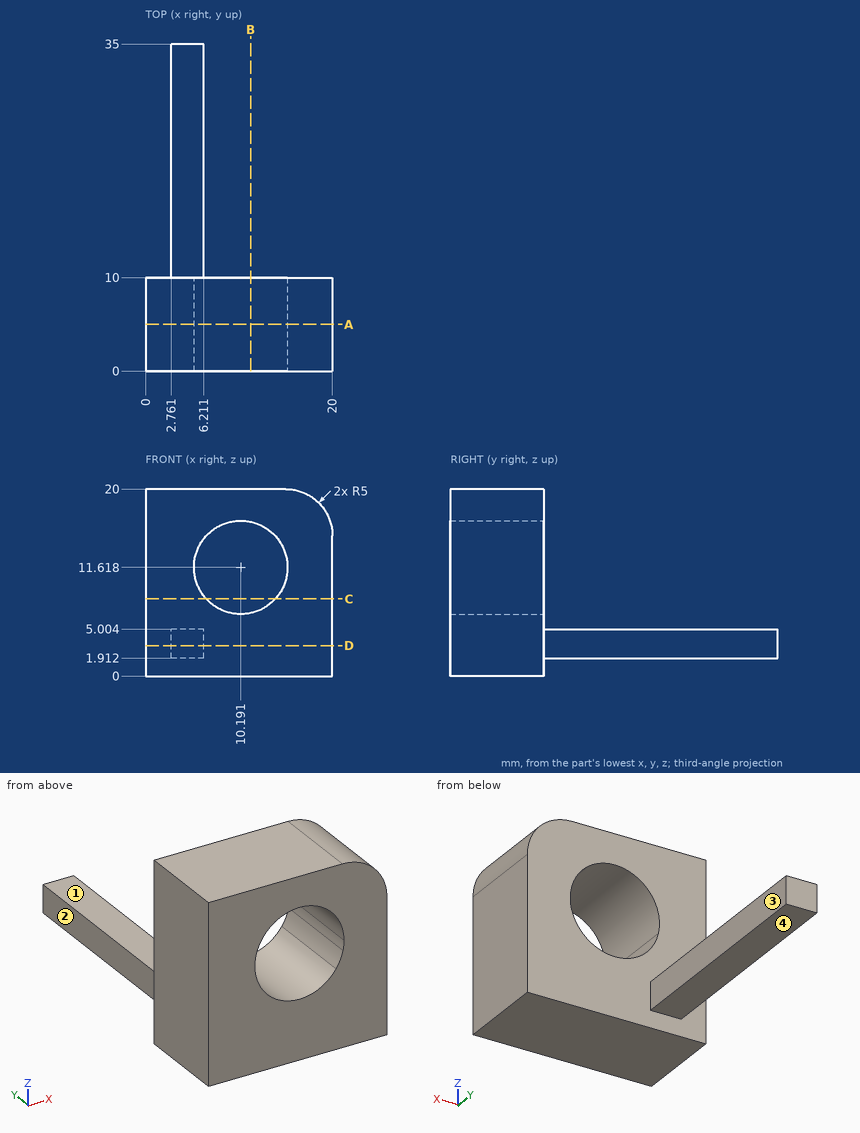
Verification items for this drawing (mm, ordinates from the low corner). A direction names the side the tool comes from. Give positions to 0.01 mm unless a question says otherwise; leave off trailing zeros. Loops run counter-clockwise (first coordinate to the right, second up) from the corner with the lowest first, then second, coordinate; pieces in that order, holes last. Notation, with made-up numbers: M -27,-27.75 L 13,-27.75 A22 ccw 13,-3.75 Z; hole C 46.5,78 d5. An arc over 180 degrees is marked long. Answer as a JSON object with one key per item and string values. Group by question number.
Item 1: Material ranges on L1, parallel to Y at x = 7, z = 3.5; L2, parallel to Z at x = 4.75, y = 22 (1 decimal); L3, parallel to X at y = 4, z = 14 (1 decimal), recorded low to high.
Item 2: Sectioned sample at D-D on z = 3.25. Record the boundary of the cut face in (x, y).
Item 3: Gauge pin test, flat ends, axial feed: pin 1 (1.5 mm diameter, centred on y = 27.5, z = 3.5, fed in from +X); pin 2 (0.9 mm diameter, centred on y = 26, z = 4, fed in from -X); pin 3 (12 mm diameter, centred on x = 9.5, z = 12.5, fed in from +Y). Record the tip position at first contact, or that the pin passes through.
Item 4: Sectioned sample at C-C on z = 8.25. Record the boundary of the cut face in (x, y) (1 decimal), plus the area to 3 significant figures.
Item 5: Access from +Z, -Z, +X, -X, +Y, -Y to the whole of each face (thin tool, end or side, straight path). Record for the marked faces 1, 2, 3 and 4.
Item 6: Sectioned sample at B-B on x = 11.25. Record the boundary of the cut face in (y, z) (1 decimal), plus the area to 3 significant figures.
Item 7: Sectioned sample at A-A on y = 5. Record the boundary of the cut face in (x, z) (1 decimal), plus the area to 3 significant figures.
Findings below:
{
 "1": {"L1": "0 to 10", "L2": "1.9 to 5", "L3": "0 to 5.8, 14.6 to 20"},
 "2": {"outline": "M 0,0 L 20,0 L 20,10 L 6.21,10 L 6.21,35 L 2.76,35 L 2.76,10 L 0,10 Z"},
 "3": {"pin 1": "x = 6.21", "pin 2": "x = 2.76", "pin 3": "y = 10"},
 "4": {"outline": "M 0,0 L 6.5,0 L 6.5,10 L 0,10 Z; M 13.9,0 L 20,0 L 20,10 L 13.9,10 Z", "area": "126 mm2"},
 "5": {"face 1": "+Z, +X, -X, +Y", "face 2": "+Z, -Z, -X, +Y", "face 3": "+Z, -Z, +X, +Y", "face 4": "-Z, +X, -X, +Y"},
 "6": {"outline": "M 0,0 L 10,0 L 10,6.7 L 0,6.7 Z; M 0,16.5 L 10,16.5 L 10,20 L 0,20 Z", "area": "102 mm2"},
 "7": {"outline": "M 0,0 L 20,0 L 20,15 A5 ccw 15,20 L 0,20 Z; hole C 10.2,11.6 d10", "area": "316 mm2"}
}
